Verification items for the finished model (mm, model axes). Face numbers are marked on the shaded views. A direction names the side the tool comes from. Coordinates: 2 decimals unless noted, no trailing zeros. Write each loop counter-clockwise with the first axis right and the second up, starting at its lowest first coordinate (ties: lowest second). Pieces come first, ordered by that corner, then holes. Notation, with made-up numbers: (39.5, 16.25) - (56.5, 16.25) arc R19 ccw to (56.5, 23.25) - close; hole circle Ø1 at (-28.5, 26). An arc over 180 degrees is marked (long way). Use one line per item in the form item = value. Start each with the question number.
(1) Sectioned sample at C-C (z = 2.5). Record the cut outline in (x, y), and give its area (3 significant figures).
(2) Gauge pin test, flat ends, axial feed: pin 1 Ø1.2 at (y, z) = (-13, 1.5) entering from -X; pin 2 Ø4.5 at (y, z) = (-12.5, 2.5) entering from +X; pin 3 Ø5 at (x, z) = (5.5, 3) entering from +Y. Record the tip position at first contact, or that the pin passes through.
(3) Material ranges on line 1 (Y direction, x = 9.5, z = 2.5); line 2 (Z direction, x = 7, y = 2); line 3 (Y direction, x = -12.5, z = 1.5), recorded low to high. Write a range as [from, to].
(4) Tool access check on the marked faces 4, 5 and 6. Record the directions out of +Z, -Z, +X, -X, +Y, -Y that give a thin tool (end or side, any length) a straight path to the whole face; none if there is none.
(5) Sectioned sample at D-D (y = 5.5). Record the cut outline in (x, z).
(6) Mould release check, pull along Y, two halves, no side actions. Record for the marked faces 1, 2 and 3: released by +Y, released by -Y, zero draft, split by the parting line, or undercut.
(7) Sectioned sample at A-A (y = 0). Record the cut outline in (x, z).
(8) Sectioned sample at B-B (x = -9.5). Record the cut outline in (y, z).
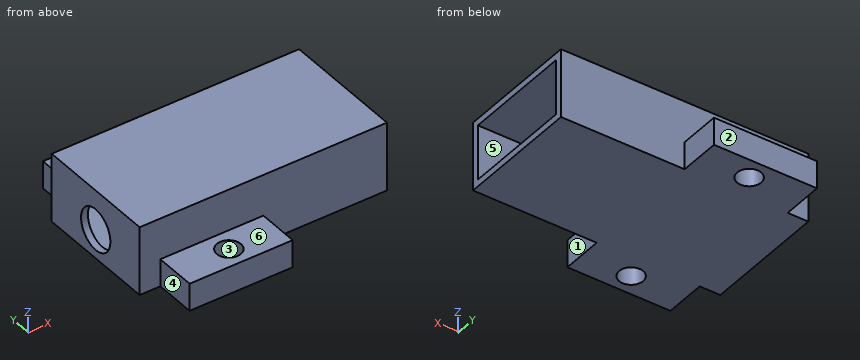
from build123d import *

# Parameters (mm, degrees)
SKETCH1_W           = 36
SKETCH1_H           = 18
BOSS_EXTRUDE1_DEPTH = 10
SHELL1_T            = -1
SKETCH2_R           = 3
CUT_EXTRUDE1_DEPTH  = 8
SKETCH3_W           = 15
SKETCH3_H           = 6
BOSS_EXTRUDE2_DEPTH = 4
SKETCH4_R           = 1.75
CUT_EXTRUDE2_DEPTH  = 12


with BuildPart() as part:
    # Sketch1 → Boss-Extrude1 (new body)
    with BuildSketch(Plane.XY):
        Rectangle(SKETCH1_W, SKETCH1_H)
    extrude(amount=BOSS_EXTRUDE1_DEPTH)

    # Shell1
    shell1_openings = [part.faces().sort_by_distance(p)[0] for p in [
        (18, 0, 5),
    ]]
    offset(amount=SHELL1_T, openings=shell1_openings, kind=Kind.INTERSECTION)

    # Sketch2 → Cut-Extrude1 (cut)
    with BuildSketch(Plane.ZY.offset(18)):
        with Locations(Location((4.221831089, 0, 0), (0, 0, 270))):
            Circle(SKETCH2_R)
    extrude(amount=-CUT_EXTRUDE1_DEPTH, mode=Mode.SUBTRACT)

    # Sketch3 → Boss-Extrude2 (add)
    with BuildSketch(Plane(origin=(0, 0, 0), x_dir=(-1, 0, 0), z_dir=(0, 0, -1))):
        with Locations((7.5, 12)):
            Rectangle(SKETCH3_W, SKETCH3_H)
        with Locations((7.5, -12)):
            Rectangle(SKETCH3_W, SKETCH3_H)
    extrude(amount=-BOSS_EXTRUDE2_DEPTH)

    # Sketch4 → Cut-Extrude2 (cut)
    with BuildSketch(Plane(origin=(0, 0, 0), x_dir=(-1, 0, 0), z_dir=(0, 0, -1))):
        with Locations((7.189144768, 12.089124741)):
            Circle(SKETCH4_R)
        with Locations((7.189144768, -12.045861265)):
            Circle(SKETCH4_R)
    extrude(amount=-CUT_EXTRUDE2_DEPTH, mode=Mode.SUBTRACT)


solid = part.part
Answers below:
q1.outline = (-18, -9) - (-15, -9) - (-15, -15) - (0, -15) - (0, -9) - (18, -9) - (18, -8) - (-17, -8) - (-17, -2.46) - (-18, -2.46) - close; (-18, 2.46) - (-17, 2.46) - (-17, 8) - (18, 8) - (18, 9) - (0, 9) - (0, 15) - (-15, 15) - (-15, 9) - (-18, 9) - close; hole circle Ø3.5 at (-7.19, -12.05); hole circle Ø3.5 at (-7.19, 12.09)
q1.area = 244 mm2
q2.pin_1 = -15
q2.pin_2 = 0
q2.pin_3 = 9
q3.line_1 = [-9, -8], [8, 9]
q3.line_2 = [0, 1], [9, 10]
q3.line_3 = [-15, -8], [8, 15]
q4.face_4 = +Z, -Z, -X, -Y
q4.face_5 = +X
q4.face_6 = +Z, +X, -X, -Y
q5.outline = (-18, 0) - (18, 0) - (18, 1) - (-17, 1) - (-17, 9) - (18, 9) - (18, 10) - (-18, 10) - close
q6.face_1 = zero draft
q6.face_2 = released by +Y
q6.face_3 = undercut
q7.outline = (-18, 0) - (18, 0) - (18, 1) - (-17, 1) - (-17, 1.22) - (-18, 1.22) - close; (-18, 7.22) - (-17, 7.22) - (-17, 9) - (18, 9) - (18, 10) - (-18, 10) - close
q8.outline = (-15, 0) - (15, 0) - (15, 4) - (9, 4) - (9, 10) - (-9, 10) - (-9, 4) - (-15, 4) - close; hole (-8, 1) - (8, 1) - (8, 9) - (-8, 9) - close
